Verification items for the finished model (mm, model axes). A direction names the side the tool comes from. Give positions to 0.01 mm unless a question says otherwise; leave off trailing zeros. Write each loop counter-clockwise with the first axis right and the second up, starting at its lowest first coordinate (ties: lowest second). Pieces come first, ordered by that corner, then holes. Notation, with made-up numbers: (45, 88) -> (94, 88) arc R5 cw to (94, 97) -> close; hole circle Ø4 at (-38, -19.75). An arc over 180 degrees is marked (long way). Use one line per item in the form item = value. Start each with the question number.
(1) Section check B-B, the plane z = 63. Record the cut outline in (x, y).
(2) Section check A-A, the plane z = 113.5. Record the cut outline in (x, y), plus the area to 3 significant figures.
(3) Depth check by flat-ended pin: pin 1 Ø8.5 at (x, z) = (26, 115.5) entering from +Y; pin 2 Ø10 at (x, y) = (-0.5, 22) entering from -Z; pin 3 Ø8.5 at (x, z) = (-26, 110.5) entering from -Y; pin 4 Ø8.5 at (y, z) = (-25.5, 111) entering from +X. Enter the tip coordinate at first touch or a pass-through.
(4) Section check C-C, the plane z = 45.5. Record the cut outline in (x, y), plus the area to 3 significant figures.
(5) Set-up check for faces 1 (the face through (-27.94, -24, 112)), 2 (the face through (-24, 20.32, 112)), 3 (the face through (27.94, 24, 112)): record each of +Z, -Z, +X, -X, +Y, -Y from which the full face is reachable in a straight line by a thin tool's end or side.
(6) Scan lines: L1, parallel to Z at x = -10, y = -2; L2, parallel to Z at x = 11.5, y = 12.5; L3, parallel to X at y = -37, z = 82. Record each from-to range of solid material in increasing order.
(7) Release check for a two-part mould opening along X. For faces 4 (the face through (-20.32, 24, 112)), 5 (the face through (-43.256, 18.212, 70.978)), 6 (the face through (-24, -27.94, 112)) record: pulls with the +X half, pulls with the -X half, needs draft (parallel to the pull), parting line crosses it, or undercut.
from build123d import *

# Parameters (mm, degrees)
F2_DEPTH  = 60.96
F4_DEPTH  = 20.32
F9_W      = 7.62
F9_H      = 7.62
F14_DEPTH = 20.32


with BuildPart() as f2:
    # F0 (on Top) → F2 (new body)
    with BuildSketch(Plane.XY):
        Polygon((35.9210244843, 35.9210244843), (0, 50.8), (0, -50.8), (35.9210244843, -35.9210244843), (50.8, 0), align=None)
    extrude(amount=F2_DEPTH)

    # F3 (on offset) → F4 (join)
    with BuildSketch(Plane.XY.offset(60.96)):
        Polygon((35.9210244843, 35.9210244843), (0, 50.8), (-35.9210244843, 35.9210244843), (-50.8, 0), (-35.9210244843, -35.9210244843), (0, -50.8), (35.9210244843, -35.9210244843), (50.8, 0), align=None)
    extrude(amount=F4_DEPTH)

    # F7 (on offset) → F13 section 0
    with BuildSketch(Plane.XY.offset(81.28)):
        Polygon((0, 50.8), (-35.9210244843, 35.9210244843), (-50.8, 0), (-35.9210244843, -35.9210244843), (0, -50.8), (35.9210244843, -35.9210244843), (50.8, 0), (35.9210244843, 35.9210244843), align=None)
    # F8 (on offset) → F13 section 1
    with BuildSketch(Plane.XY.offset(101.6)):
        Polygon((43.1052293811, 0), (30.48, 30.48), (0, 43.1052293811), (-30.48, 30.48), (-43.1052293811, 0), (-30.48, -30.48), (0, -43.1052293811), (30.48, -30.48), align=None)
    loft()

    # F9 (on offset) → F14 (join)
    with BuildSketch(Plane.XY.offset(101.6)):
        with Locations((-24.13, 24.13)):
            Rectangle(F9_W, F9_H)
        with Locations((24.13, 24.13)):
            Rectangle(F9_W, F9_H)
        with Locations((-24.13, -24.13)):
            Rectangle(F9_W, F9_H)
        with Locations((24.13, -24.13)):
            Rectangle(F9_W, F9_H)
    extrude(amount=F14_DEPTH)

    # F15 (on Front) → F16 (revolve)
    with BuildSketch(Plane.XZ):
        with BuildLine():
            ThreePointArc((0, 160.02), (-30.0961069105, 149.4685742909), (-46.1642209939, 121.92))
            Line((-46.1642209939, 121.92), (0, 121.92))
            Line((0, 121.92), (0, 160.02))
        make_face()
    revolve(axis=Axis((0, 0, 140.97), (0, 0, 1)))


solid = f2.part
Completed:
q1.outline = (-50.8, 0) -> (-35.92, -35.92) -> (0, -50.8) -> (35.92, -35.92) -> (50.8, 0) -> (35.92, 35.92) -> (0, 50.8) -> (-35.92, 35.92) -> close
q2.outline = (-27.94, -27.94) -> (-20.32, -27.94) -> (-20.32, -20.32) -> (-27.94, -20.32) -> close; (-27.94, 20.32) -> (-20.32, 20.32) -> (-20.32, 27.94) -> (-27.94, 27.94) -> close; (20.32, -27.94) -> (27.94, -27.94) -> (27.94, -20.32) -> (20.32, -20.32) -> close; (20.32, 20.32) -> (27.94, 20.32) -> (27.94, 27.94) -> (20.32, 27.94) -> close
q2.area = 232 mm²
q3.pin_1 = 27.94
q3.pin_2 = 0
q3.pin_3 = -27.94
q3.pin_4 = 27.94
q4.outline = (0, -50.8) -> (35.92, -35.92) -> (50.8, 0) -> (35.92, 35.92) -> (0, 50.8) -> close
q4.area = 3,650 mm²
q5.face_1 = -X, +Y, -Y
q5.face_2 = +X, -X
q5.face_3 = +X, +Y, -Y
q6.L1 = 60.96 to 101.6, 121.92 to 159.04
q6.L2 = 0 to 101.6, 121.92 to 157.06
q6.L3 = -32.66 to 32.66
q7.face_4 = undercut
q7.face_5 = pulls with the -X half
q7.face_6 = needs draft
